Check sheet for the modelled part. Datum: model origin and axes. Units: mm. A direction names the side the tool comes from. Coordinates: 2 decimals unless noted, no trailing zeros. Loops run counter-clockwise (first coordinate to the right, second up) from the corner with the lowest first, then second, coordinate; pieces in that order, holes last.
```python
from build123d import *

# Parameters (mm, degrees)
SKETCH_R     = 12.5
PAD_DEPTH    = 25
SKETCH001_R  = 16.5
PAD001_DEPTH = 5
SKETCH002_R  = 13
PAD002_DEPTH = 2
FILLET_R     = 2
FILLET001_R  = 0.5


with BuildPart() as part:
    # Sketch → Pad (new body)
    with BuildSketch(Plane.XY):
        Circle(SKETCH_R)
    extrude(amount=PAD_DEPTH)

    # Sketch001 (on Face3 of Pad) → Pad001 (join)
    with BuildSketch(Plane.XY.offset(25)):
        Circle(SKETCH001_R)
    extrude(amount=PAD001_DEPTH)

    # Sketch002 (on Face3 of Pad001) → Pad002 (join)
    with BuildSketch(Plane.XY.offset(30)):
        Circle(SKETCH002_R)
    extrude(amount=PAD002_DEPTH)

    # Fillet
    fillet_edges = [part.edges().sort_by_distance(p)[0] for p in [
        (-16.5, 0, 30),
    ]]
    fillet(fillet_edges, radius=FILLET_R)

    # Fillet001
    fillet001_edges = [part.edges().sort_by_distance(p)[0] for p in [
        (-13, 0, 32),
    ]]
    fillet(fillet001_edges, radius=FILLET001_R)


solid = part.part
```
1) Section check C-C on z = 20. Enter the section's corners in (x, y), plus the area to 3 significant figures.
Answer sheet:
outline: circle Ø25 at (0, 0)
area: 491 mm2
2) Depth check by flat-ended pin: pin 1 (1 mm diameter, centred on y = -3.5, z = 13, fed in from +X); pin 2 (6 mm diameter, centred on y = 3.5, z = 14.5, fed in from -X); pin 3 (2 mm diameter, centred on y = -1, z = 28.5, fed in from -X). Enter the tip coordinate at first touch or a pass-through.
Answer sheet:
pin 1: stops at x = 12.13
pin 2: stops at x = -12.49
pin 3: stops at x = -16.5
3) Section check A-A on x = 0. Enter the section's corners in (y, z).
Answer sheet:
outline: (-16.5, 25) - (-12.5, 25) - (-12.5, 0) - (12.5, 0) - (12.5, 25) - (16.5, 25) - (16.5, 28) arc R2 ccw to (14.5, 30) - (13, 30) - (13, 31.5) arc R0.5 ccw to (12.5, 32) - (-12.5, 32) arc R0.5 ccw to (-13, 31.5) - (-13, 30) - (-14.5, 30) arc R2 ccw to (-16.5, 28) - close
4) Scan lines: line 1 (Z direction, x = -3, y = -13); line 2 (X direction, y = 1.5, z = 18.5); line 3 (Y direction, x = -6, z = 27). Record each from-to range of solid material in increasing order.
Answer sheet:
line 1: z = 25 to 30
line 2: x = -12.41 to 12.41
line 3: y = -15.37 to 15.37
5) Section check D-D on z = 26. Enter the section's corners in (x, y), plus the area to 3 significant figures.
Answer sheet:
outline: circle Ø33 at (0, 0)
area: 855 mm2
6) Mould release check, pull along Z, two halves, no side actions. Record for faces 3 (the flat face through (-9, 10, 30)), 4 (the cylindrical face through (11.923, 3.755, 12.325)), 5 (the flat face through (-12.3, 3.7, 25)): +Z half, -Z half, draft (parallel to the pull), parting line (faces both ways), or undercut.
Answer sheet:
face 3: +Z half
face 4: draft
face 5: -Z half
7) Set-up check for faces 1 (the cylindrical face through (15.24, -6.32, 26.48)), 2 (the cylindrical face through (-10.316, -7.91, 30.74)): record each of +Z, -Z, +X, -X, +Y, -Y from which the full face is reachable in a straight line by a thin tool's end or side.
Answer sheet:
face 1: +Z, -Z
face 2: +Z
